The model under review builds one solid part; all positions refer to its coordinate system, in mm. A direction names the side the tool comes from. Coordinates: 2 decimals unless noted, no trailing zeros. Loops run counter-clockwise (first coordinate to the right, second up) from the corner with the lowest first, then second, coordinate; pieces in that order, holes last. Notation, with made-up numbers: M 87,-3 L 124,-3 A36 cw 124,32 Z; hole C 24,4 d3. An arc over 180 degrees is marked long. Write item = value, one per line. Start each with the question number.
Q1. We need section C-C on z = 9. Give the boundary of the cut face in (x, y).
Q2. We need section D-D on z = 13. Give the boundary of the cut face in (x, y).
Q3. We need section A-A on x = 0. Give the boundary of the cut face in (y, z).
Q4. Wall thickness on probe 1 along Z at (x, y) = (49.5, 5.5); probe 2 along X at (y, z) = (-5.75, 3.5); probe 3 along X at (y, z) = (8.5, 4.25): over which ranges is each line inside the solid? List them lowest first.
Q5. For faces 1 (the face through (-10, 0, 2)), 2 (the face through (-1.08, -4.88, 7.46)), list the 3-axis set-ups (+Z, -Z, +X, -X, +Y, -Y) from which the entire face can be reached by the end or side of a thin tool; tool diameter is ignored.
Q6. Clearance check with flat-ended pins moving along their axes: pin 1 Ø1 at (x, y) = (40.5, 2) entering from +Z; pin 2 Ø1.5 at (y, z) = (4, 11.5) entering from -X; pin 3 Ø3 at (y, z) = (1.5, 11) entering from +X. State where each tip first meets the part, or that it passes through.
Q7. We need section B-B on y = 0. Give the boundary of the cut face in (x, z), and give its area (3 significant figures).
from build123d import *

# Parameters (mm, degrees)
F0_W     = 100
F0_H     = 20
F1_DEPTH = 5
F2_R     = 5
F3_DEPTH = 10
F4_R     = 5
F5_R     = 5


with BuildPart() as f1:
    # F0 (on Top) → F1 (new body)
    with BuildSketch(Plane.XY):
        with Locations((40, 0)):
            Rectangle(F0_W, F0_H)
    extrude(amount=F1_DEPTH)

    # F2 (on face) → F3 (join)
    with BuildSketch(Plane.XY.offset(5)):
        Circle(F2_R)
    extrude(amount=F3_DEPTH)

    # F4
    f4_edges = [f1.edges().sort_by_distance(p)[0] for p in [
        (-10, -10, 2.5),
        (-10, 10, 2.5),
    ]]
    fillet(f4_edges, radius=F4_R)

    # F5
    f5_edges = [f1.edges().sort_by_distance(p)[0] for p in [
        (-5, 0, 15),
    ]]
    fillet(f5_edges, radius=F5_R)


solid = f1.part
Returned:
q1.outline = C 0,0 d10
q2.outline = C 0,0 d8
q3.outline = M -10,0 L 10,0 L 10,5 L 5,5 L 5,10 A5 ccw -5,10 L -5,5 L -10,5 Z
q4.probe_1 = 0 to 5
q4.probe_2 = -9.94 to 90
q4.probe_3 = -8.57 to 90
q5.face_1 = +Z, -Z, -X, +Y, -Y
q5.face_2 = +Z
q6.pin_1 = 5
q6.pin_2 = -3.55
q6.pin_3 = 4.99
q7.outline = M -10,0 L 90,0 L 90,5 L 5,5 L 5,10 A5 ccw -5,10 L -5,5 L -10,5 Z
q7.area = 589 mm^2
